from build123d import *

# Parameters (mm, degrees)
SKETCH1_W           = 79
SKETCH1_H           = 110
SKETCH1_R           = 16
SKETCH1_R_2         = 11
SKETCH1_R_3         = 2.1
SKETCH1_R_4         = 1.25
BOSS_EXTRUDE1_DEPTH = 2.5
SKETCH2_R           = 2.5
CUT_EXTRUDE1_DEPTH  = 648.672345596
FILLET1_R           = 10
FILLET2_R           = 5


with BuildPart() as part:
    # Sketch1 → Boss-Extrude1 (new, symmetric)
    with BuildSketch(Plane.XY):
        Rectangle(SKETCH1_W, SKETCH1_H)
        with Locations((0, -25)):
            Circle(SKETCH1_R, mode=Mode.SUBTRACT)
        with Locations((0, 33.6)):
            Circle(SKETCH1_R_2, mode=Mode.SUBTRACT)
        with Locations((21, -25)):
            Circle(SKETCH1_R_3, mode=Mode.SUBTRACT)
        with Locations((-21, -25)):
            Circle(SKETCH1_R_3, mode=Mode.SUBTRACT)
        with Locations((0, -4)):
            Circle(SKETCH1_R_3, mode=Mode.SUBTRACT)
        with Locations((0, -46)):
            Circle(SKETCH1_R_3, mode=Mode.SUBTRACT)
        with Locations((15.5, 49.1)):
            Circle(SKETCH1_R_4, mode=Mode.SUBTRACT)
        with Locations((15.5, 18.1)):
            Circle(SKETCH1_R_4, mode=Mode.SUBTRACT)
        with Locations((-15.5, 18.1)):
            Circle(SKETCH1_R_4, mode=Mode.SUBTRACT)
        with Locations((-15.5, 49.1)):
            Circle(SKETCH1_R_4, mode=Mode.SUBTRACT)
        with Locations((-17, 7.5)):
            Circle(SKETCH1_R_3, mode=Mode.SUBTRACT)
        with Locations((9.941037343, 0)):
            Circle(SKETCH1_R_3, mode=Mode.SUBTRACT)
        with Locations((31, -25)):
            Circle(SKETCH1_R_3, mode=Mode.SUBTRACT)
        with Locations((-9.466357856, -50.166900153)):
            Circle(SKETCH1_R_3, mode=Mode.SUBTRACT)
        with Locations((-31, -25)):
            Circle(SKETCH1_R_3, mode=Mode.SUBTRACT)
        with BuildLine():
            Line((7.5, 11.6), (19.5, 11.6))
            ThreePointArc((19.5, 11.6), (22, 9.1), (19.5, 6.6))
            Line((19.5, 6.6), (7.5, 6.6))
            ThreePointArc((7.5, 6.6), (5, 9.1), (7.5, 11.6))
        make_face(mode=Mode.SUBTRACT)
    extrude(amount=BOSS_EXTRUDE1_DEPTH, both=True)

    # Sketch2 → Cut-Extrude1 (cut, through all)
    with BuildSketch(Plane(origin=(-158.166263917, -561.751583183, 2.5), x_dir=(1, 0, 0), z_dir=(0, 0, 1))):
        with Locations((136.066263917, 558.251583183)):
            Circle(SKETCH2_R)
        with Locations(Location((180.666263917, 558.251583183, 0), (0, 0, 180))):
            Circle(SKETCH2_R)
        with Locations(Location((136.066263917, 515.251583183, 0), (0, 0, 180))):
            Circle(SKETCH2_R)
        with Locations((180.666263917, 515.251583183)):
            Circle(SKETCH2_R)
        with BuildLine():
            Line((191.966263917, 559.251583183), (191.966263917, 557.251583183))
            ThreePointArc((191.966263917, 557.251583183), (190.666263917, 555.951583183), (189.366263917, 557.251583183))
            Line((189.366263917, 557.251583183), (189.366263917, 559.251583183))
            ThreePointArc((189.366263917, 559.251583183), (190.666263917, 560.551583183), (191.966263917, 559.251583183))
        make_face()
        with BuildLine():
            Line((173.566263917, 557.251583183), (173.566263917, 559.251583183))
            ThreePointArc((173.566263917, 559.251583183), (174.866263917, 560.551583183), (176.166263917, 559.251583183))
            Line((176.166263917, 559.251583183), (176.166263917, 557.251583183))
            ThreePointArc((176.166263917, 557.251583183), (174.866263917, 555.951583183), (173.566263917, 557.251583183))
        make_face()
        with BuildLine():
            Line((142.966263917, 557.251583183), (142.966263917, 559.251583183))
            ThreePointArc((142.966263917, 559.251583183), (141.666263917, 560.551583183), (140.366263917, 559.251583183))
            Line((140.366263917, 559.251583183), (140.366263917, 557.251583183))
            ThreePointArc((140.366263917, 557.251583183), (141.666263917, 555.951583183), (142.966263917, 557.251583183))
        make_face()
        with BuildLine():
            Line((124.766263917, 559.251583183), (124.766263917, 557.251583183))
            ThreePointArc((124.766263917, 557.251583183), (126.066263917, 555.951583183), (127.366263917, 557.251583183))
            Line((127.366263917, 557.251583183), (127.366263917, 559.251583183))
            ThreePointArc((127.366263917, 559.251583183), (126.066263917, 560.551583183), (124.766263917, 559.251583183))
        make_face()
        with BuildLine():
            Line((124.566263917, 514.251583183), (124.566263917, 516.251583183))
            ThreePointArc((124.566263917, 516.251583183), (125.866263917, 517.551583183), (127.166263917, 516.251583183))
            Line((127.166263917, 516.251583183), (127.166263917, 514.251583183))
            ThreePointArc((127.166263917, 514.251583183), (125.866263917, 512.951583183), (124.566263917, 514.251583183))
        make_face()
        with BuildLine():
            Line((142.966263917, 516.251583183), (142.966263917, 514.251583183))
            ThreePointArc((142.966263917, 514.251583183), (141.666263917, 512.951583183), (140.366263917, 514.251583183))
            Line((140.366263917, 514.251583183), (140.366263917, 516.251583183))
            ThreePointArc((140.366263917, 516.251583183), (141.666263917, 517.551583183), (142.966263917, 516.251583183))
        make_face()
        with BuildLine():
            Line((173.366263917, 516.251583183), (173.366263917, 514.251583183))
            ThreePointArc((173.366263917, 514.251583183), (174.666263917, 512.951583183), (175.966263917, 514.251583183))
            Line((175.966263917, 514.251583183), (175.966263917, 516.251583183))
            ThreePointArc((175.966263917, 516.251583183), (174.666263917, 517.551583183), (173.366263917, 516.251583183))
        make_face()
        with BuildLine():
            Line((191.966263917, 514.251583183), (191.966263917, 516.251583183))
            ThreePointArc((191.966263917, 516.251583183), (190.666263917, 517.551583183), (189.366263917, 516.251583183))
            Line((189.366263917, 516.251583183), (189.366263917, 514.251583183))
            ThreePointArc((189.366263917, 514.251583183), (190.666263917, 512.951583183), (191.966263917, 514.251583183))
        make_face()
    extrude(amount=-CUT_EXTRUDE1_DEPTH, mode=Mode.SUBTRACT)

    # Fillet1
    fillet1_edges = [part.edges().sort_by_distance(p)[0] for p in [
        (-39.5, 55, 0),
        (39.5, 55, 0),
    ]]
    fillet(fillet1_edges, radius=FILLET1_R)

    # Fillet2
    fillet2_edges = [part.edges().sort_by_distance(p)[0] for p in [
        (39.5, -55, 0),
        (-39.5, -55, 0),
    ]]
    fillet(fillet2_edges, radius=FILLET2_R)


solid = part.part
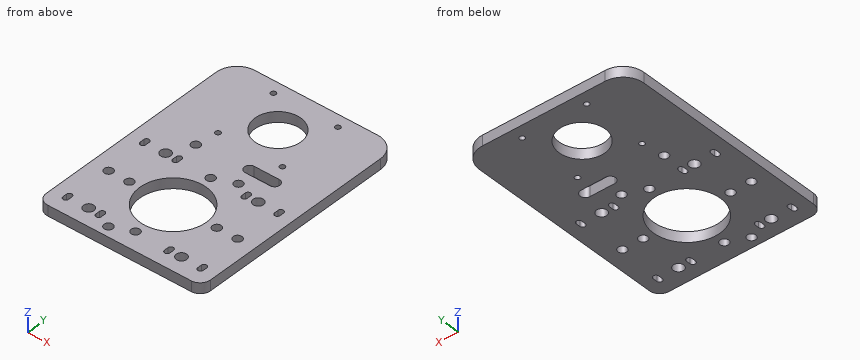
Check sheet for the modelled part. Datum: model origin and axes. Units: mm. Give positions to 0.01 mm unless a question says otherwise; leave off trailing zeros. Order: outer loops, then holes, each group sorted by start corner. A loop starts at its lowest first (then second) coordinate and runs counter-clockwise, first axis right, second up. Notation, with made-up numbers: (-37, 69.5) - (-16, 69.5) arc R19 cw to (-16, 85.5) - close; hole circle Ø7 at (78, -31.75). An arc over 180 degrees is marked (long way). Answer as CSV lines item,"result".
1. Scan lines: probe 1 along Y at (x, z) = (0, -0.6); probe 2 along Y at (x, z) = (14, -1.45); probe 3 along X at (y, z) = (-23.5, -0.7). Record each from-to range of solid material in increasing order. Write a range as from..to.
Result sheet:
probe 1,"-55..-48.1, -43.9..-41, -9..-6.1, -1.9..22.6, 44.6..55"
probe 2,"-55..-32.75, -17.25..6.6, 11.6..55"
probe 3,"-39.5..-32.47, -29.53..-22.47, -19.53..-15.93, 15.93..19.53, 22.47..29.53, 32.47..39.5"
2. Section check B-B (x = -21). Record the boundary of the cut face in (y, z) (3 decimals).
Result sheet:
outline,"(-55, -2.5) - (-48.745, -2.5) - (-48.745, 2.5) - (-55, 2.5) - close; (-44.255, -2.5) - (-27.1, -2.5) - (-27.1, 2.5) - (-44.255, 2.5) - close; (-22.9, -2.5) - (-5.745, -2.5) - (-5.745, 2.5) - (-22.9, 2.5) - close; (-1.255, -2.5) - (55, -2.5) - (55, 2.5) - (-1.255, 2.5) - close"
3. Section check D-D (z = -0.3). State how many separate pieces and enclosed holes the cut face has, then the cut area to 3 significant figures.
Result sheet:
separate pieces,"1"
enclosed holes,"28"
area,"7,070 mm²"
4. Go/stop test with a flat-tipped pin: P1, Ø4, axis at x = -15.5, y = 49.1, coming from the -Z side. Record where the tip stops, or that it passes through.
Result sheet:
P1,"z = -2.5"
5. Section check C-C (y = 49.1). Record the boundary of the cut face in (x, z).
Result sheet:
outline,"(-38.62, -2.5) - (-16.75, -2.5) - (-16.75, 2.5) - (-38.62, 2.5) - close; (-14.25, -2.5) - (14.25, -2.5) - (14.25, 2.5) - (-14.25, 2.5) - close; (16.75, -2.5) - (38.62, -2.5) - (38.62, 2.5) - (16.75, 2.5) - close"
6. Section check A-A (y = 37.5). Record the boundary of the cut face in (x, z), then the cut area to 3 significant figures.
Result sheet:
outline,"(-39.5, -2.5) - (-10.29, -2.5) - (-10.29, 2.5) - (-39.5, 2.5) - close; (10.29, -2.5) - (39.5, -2.5) - (39.5, 2.5) - (10.29, 2.5) - close"
area,"292 mm²"
